Part model, mm, in its own coordinate system. A direction names the side the tool comes from. Give positions to 0.01 mm unless a question says otherwise; leave off trailing zeros. Loops run counter-clockwise (first coordinate to the right, second up) from the corner with the lowest first, then second, coordinate; pieces in that order, holes last. Notation, with made-up numbers: M 78,69.5 L 113,69.5 A14 cw 113,96.5 Z; hole C 67,-12.5 d7. An arc over 180 degrees is marked long. Put each result on its own line as item: value. Start each with the question number.
```python
from build123d import *

# Parameters (mm, degrees)
SKETCH1_W                  = 304.8
SKETCH1_H                  = 304.8
BLANK_DEPTH                = 50.8
SKETCH2_W                  = 228.6
SKETCH2_H                  = 203.2
ROUGH_BATTERY_CAVITY_DEPTH = 41.275
SKETCH3_W                  = 304.8
SKETCH3_H                  = 15.875
BUMPER_RAIL_DEPTH          = 38.1
SKETCH4_R                  = 3.302
BUMPER_RAIL_HOLES_DEPTH    = 219.867836833
DRIVE_MOTOR_RAIL_DEPTH     = 31.75


with BuildPart() as part:
    # Sketch1 → Blank (new body)
    with BuildSketch(Plane.XY):
        Rectangle(SKETCH1_W, SKETCH1_H)
    extrude(amount=BLANK_DEPTH)

    # Sketch2 → Rough battery cavity (cut)
    with BuildSketch(Plane.XY.offset(50.8)):
        with Locations((0, -25.4)):
            Rectangle(SKETCH2_W, SKETCH2_H)
    extrude(amount=-ROUGH_BATTERY_CAVITY_DEPTH, mode=Mode.SUBTRACT)

    # Sketch3 → Bumper rail (cut)
    with BuildSketch(Plane.XY.offset(50.8)):
        with Locations((0, -144.4625)):
            Rectangle(SKETCH3_W, SKETCH3_H)
    extrude(amount=-BUMPER_RAIL_DEPTH, mode=Mode.SUBTRACT)

    # Sketch4 → Bumper rail holes (cut, through all)
    with BuildSketch(Plane.XY.offset(12.7)):
        with Locations((-127, -146.05)):
            Circle(SKETCH4_R)
        with Locations((127, -146.05)):
            Circle(SKETCH4_R)
        with Locations((-63.5, -146.05)):
            Circle(SKETCH4_R)
        with Locations((0, -146.05)):
            Circle(SKETCH4_R)
        with Locations((63.5, -146.05)):
            Circle(SKETCH4_R)
    extrude(amount=-BUMPER_RAIL_HOLES_DEPTH, mode=Mode.SUBTRACT)

    # Sketch5 → Drive motor rail (cut)
    with BuildSketch(Plane(origin=(152.4, 0, 0), x_dir=(0, 0, -1), z_dir=(1, 0, 0))):
        Polygon((-50.8, 45.440951562), (0, -63.5), (0, 96.240951562), (-50.8, 96.240951562), align=None)
        Polygon((-50.8, 7.877501429), (0, -101.063450133), (0, -126.463450133), (-50.8, -126.463450133), align=None)
    drive_motor_rail = extrude(amount=-DRIVE_MOTOR_RAIL_DEPTH, mode=Mode.SUBTRACT)

    # Drive motor rail mirror: Drive motor rail across plane
    add(drive_motor_rail.mirror(Plane(origin=(0, 0, 0), x_dir=(0, 0, 1), z_dir=(1, 0, 0))), mode=Mode.SUBTRACT)


solid = part.part
```
1) Band-saw the part on A-A on z = 39. Give the cut face in (x, y) (3 decimals), then the cut area to 3 significant figures.
2) Pin check, flat tips, straight feed: pin 1 Ø2 at (y, z) = (83.5, 7.5) entering from +X; pin 2 Ø16 at (x, z) = (131, 31) entering from -Y (3 decimals); pin 3 Ø4 at (x, y) = (-57, -57) entering from +Z (3 decimals). Stop position of each tip, or through.
3) Wall check: L1, parallel to X at y = -146, z = 2; L2, parallel to X at y = -89, z = 39.5; L3, parallel to Y at x = -111, z = 11.5. Give the ranges that are in metal, low to high.
4) Band-saw the part on B-B on x = -35. Give the cut face in (y, z) (3 decimals).
5) Band-saw the part on C-C on y = -88.5. Give the cut face in (x, z) (3 decimals).
6) Which spindle directions (+Z, -Z, +X, -X, +Y, -Y) get a long thin tool onto all of the face, cutting with end or side? Do faces 1 (the flat face through (-114.3, -27, 30)), 2 (the flat face through (-2, -143, 12.7)), 3 (the flat face through (-136.747, -8.267, 25.756)), 4 (the flat face through (137, 96.241, 25)), 5 (the flat face through (-120.65, -73, 31)). Say none if no direction does.
7) Mould opens along Y. For faces 6 (the flat face through (-2, -152.4, 6)), 7 (the flat face through (136.747, -8.267, 25.756)), 8 (the flat face through (-2, 152.4, 25)) say: +Y half, -Y half, draft (parallel to the pull), parting line (faces both ways), or undercut.
Evaluation:
1. outline: M -152.4,-136.525 L 152.4,-136.525 L 152.4,-126.463 L 120.65,-126.463 L 120.65,-17.428 L 152.4,-17.428 L 152.4,20.136 L 120.65,20.136 L 120.65,96.241 L 152.4,96.241 L 152.4,152.4 L -152.4,152.4 L -152.4,96.241 L -120.65,96.241 L -120.65,20.136 L -152.4,20.136 L -152.4,-17.428 L -120.65,-17.428 L -120.65,-126.463 L -152.4,-126.463 Z; hole M -114.3,-127 L 114.3,-127 L 114.3,76.2 L -114.3,76.2 Z
1. area: 29,900 mm2
2. pin 1: x = 120.65
2. pin 2: y = -136.525
2. pin 3: z = 9.525
3. L1: -152.4 to -130.3, -123.7 to -66.8, -60.2 to -3.3, 3.3 to 60.2, 66.8 to 123.7, 130.3 to 152.4
3. L2: -120.65 to -114.3, 114.3 to 120.65
3. L3: -152.4 to -127, 76.2 to 152.4
4. outline: M -152.4,0 L 152.4,0 L 152.4,50.8 L 76.2,50.8 L 76.2,9.525 L -127,9.525 L -127,50.8 L -136.525,50.8 L -136.525,12.7 L -152.4,12.7 Z
5. outline: M -152.4,0 L 152.4,0 L 152.4,5.858 L 120.65,5.858 L 120.65,50.8 L 114.3,50.8 L 114.3,9.525 L -114.3,9.525 L -114.3,50.8 L -120.65,50.8 L -120.65,5.858 L -152.4,5.858 Z
6. face 1: +Z
6. face 2: +Z, +X, -X, -Y
6. face 3: -Z, -X
6. face 4: +Z, -Z, +X
6. face 5: +Z, -X
7. face 6: -Y half
7. face 7: undercut
7. face 8: +Y half
